Solid Edge part; units mm, degrees
sketch "Sketch1" plane through (0, 0, 0) normal (0, 0, -1) x (-1, 0, 0)
  line L0 (-66.5566, 13.1686) -> (-55.0566, 13.1686)
  line L1 (-55.0566, 13.1686) -> (-55.0566, 22.6686)
  line L2 (-55.0566, 22.6686) -> (-66.5566, 22.6686)
  line L3 (-66.5566, 22.6686) -> (-66.5566, 13.1686)
  line L4 (-51.5566, 13.1686) -> (-40.0566, 13.1686)
  line L5 (-40.0566, 13.1686) -> (-40.0566, 22.6686)
  line L6 (-40.0566, 22.6686) -> (-51.5566, 22.6686)
  line L7 (-51.5566, 22.6686) -> (-51.5566, 13.1686)
  line L8 (-32.5566, 10.1686) -> (-18.5566, 10.1686)
  line L9 (-18.5566, 10.1686) -> (-18.5566, 22.6686)
  line L10 (-18.5566, 22.6686) -> (-36.5566, 22.6686)
  line L11 (-36.5566, 22.6686) -> (-36.5566, 12.1686)
  line L12 (-32.5566, 10.1686) -> (-36.5566, 12.1686)
  line L13 (-92.5566, 26.1578) -> (-21.5566, 26.1578)
  line L14 (-21.5566, 26.1578) -> (-15.0566, 29.1686)
  line L15 (-15.0566, 29.1686) -> (-0.0566, 29.1686)
  line L16 (-0.0566, 29.1686) -> (-0.0566, 23.1686)
  line L17 (-15.0566, 23.1686) -> (-0.0566, 23.1686)
  line L18 (-15.0566, 23.1686) -> (-15.0566, 12.6686)
  line L19 (-15.0566, 12.6686) -> (-0.0566, 12.6686)
  line L20 (-0.0566, 12.6686) -> (-0.0566, 2.6686)
  line L21 (-26.2997, 2.6686) -> (-0.0566, 2.6686)
  line L22 (-40.1546, 9.1578) -> (-26.2997, 2.6686)
  line L23 (-65.1546, 9.1578) -> (-40.1546, 9.1578)
  line L24 (-77.5566, -0.3422) -> (-65.1546, 9.1578)
  line L25 (-92.5566, -0.3422) -> (-77.5566, -0.3422)
  line L26 (-92.5566, 3.6578) -> (-92.5566, -0.3422)
  line L27 (-92.5566, 3.6578) -> (-78.5566, 3.6578)
  line L28 (-78.5566, 3.6578) -> (-71.5566, 9.1578)
  line L29 (-92.5566, 9.1578) -> (-71.5566, 9.1578)
  line L30 (-92.5566, 9.1578) -> (-92.5566, 13.1578)
  line L31 (-92.5566, 13.1578) -> (-70.0566, 13.1578)
  line L32 (-70.0566, 13.1578) -> (-70.0566, 22.1578)
  line L33 (-92.5566, 22.1578) -> (-70.0566, 22.1578)
  line L34 (-92.5566, 22.1578) -> (-92.5566, 26.1578)
  dimension "D1" = 0.0566
  dimension "D2" = 15.0566
  dimension "D3" = 15.0566
  dimension "D4" = 0.0566
  dimension "D5" = 92.5566
  dimension "D6" = 66.5566
  dimension "D7" = 55.0566
  dimension "D8" = 70.0566
  dimension "D9" = 92.5566
  dimension "D10" = 92.5566
  dimension "D11" = 92.5566
  dimension "D12" = 40.1546
  dimension "D13" = 32.5566
  dimension "D14" = 18.5566
  dimension "D15" = 18.5566
  dimension "D16" = 36.5566
  dimension "D17" = 32.5566
  dimension "D18" = 92.5566
  dimension "D19" = 15.0566
  dimension "D20" = 26.2997
  dimension "D21" = 65.1546
  dimension "D22" = 92.5566
  dimension "D23" = 92.5566
  dimension "D24" = 92.5566
  dimension "D25" = 77.5566
extrude "Protrusion1" add sketch "Sketch1" against normal blind 15.0368
sketch "Sketch2" plane through (13.1782, 2.6686, 7.5184) normal (0, -1, 0) x (1, 0, 0)
  line L0 (74.2537, 1.7409) -> (1.8784, 6.3912)
extrude "Enlèvement_matière_1" cut sketch "Sketch2" along normal mid plane 64.6684 material side at (51.2475, 2.6686, 11.6343)
sketch "Sketch3" plane through (7.6241, 29.1686, 7.4367) normal (0, 1, 0) x (-1, 0, 0)
  circle A0 centre (0.0398, 0.1367) radius 2.0955
  circle A1 centre (-79.9299, -2.362) radius 2.1098
extrude "Enlèvement_matière_3" cut sketch "Sketch3" along normal mid plane 246.888
fillet "Congé_1" radius 7.1911 4 edges at (0.0566, 26.1686, 14.8734) (0.0566, 7.6686, 14.8734) (0.0566, 26.1686, 0) (0.0566, 7.6686, 0)
fillet "Congé_2" radius 4.5761 6 edges at (92.5566, 1.6578, 8.93) (92.5566, 11.1578, 8.93) (92.5566, 24.1578, 8.93) (92.5566, 24.1578, 0) (92.5566, 11.1578, 0) (92.5566, 1.6578, 0)
fillet "Congé_3" radius 2.0593 15 edges at (15.0566, 23.1686, 6.9548) (15.0566, 12.6686, 6.9548) (36.5566, 22.6686, 6.2641) (36.5566, 12.1686, 6.2641) (32.5566, 10.1686, 6.3926) (18.5566, 10.1686, 6.8424) (18.5566, 22.6686, 6.8424) (40.0566, 13.1686, 6.1516) (40.0566, 22.6686, 6.1516) (51.5566, 22.6686, 5.7822) (55.0566, 13.1686, 5.6697) (51.5566, 13.1686, 5.7822) (55.0566, 22.6686, 5.6697) (66.5566, 22.6686, 5.3003) (66.5566, 13.1686, 5.3003)
fillet "Congé_5" radius 2.0593 2 edges at (70.0566, 13.1578, 5.1878) (70.0566, 22.1578, 5.1878)
fillet "Congé_6" radius 1.0296 2 edges at (71.5566, 9.1578, 5.1397) (78.5566, 3.6578, 4.9148)
fillet "Congé_7" radius 6.35 1 edges at (77.5566, -0.3422, 4.9469)
fillet "Congé_8" radius 6.35 5 edges at (40.1546, 9.1578, 6.1485) (65.1546, 9.1578, 5.3453) (26.2997, 2.6686, 6.5936) (15.0566, 29.1686, 6.9548) (21.5566, 26.1578, 6.746)
sketch "Sketch4" plane through (12.4715, 2.6686, 7.1983) normal (0, -1, 0) x (1, 0, 0)
  line L0 (-4.4993, -3.3547) -> (9.8456, -1.8628)
  line L1 (-4.03, 4.0259) -> (9.569, 2.6247)
  arc A0 (-4.03, 4.0259) -> (-4.4993, -3.3547) centre (-4.8872, 0.3752) ccw
  arc A1 (9.8456, -1.8628) -> (9.569, 2.6247) centre (9.6128, 0.3752) ccw
extrude "Enlèvement_matière_4" cut sketch "Sketch4" against normal blind 5.498
properties part number "AC_1.04"
Design review of the part built by this model. Coordinates are the model's own, in mm. A direction names the side the tool comes from. Coordinates: 2 decimals unless noted, no trailing zeros. Loops run counter-clockwise (first coordinate to the right, second up) from the corner with the lowest first, then second, coordinate; pieces in that order, holes last.
Item 1: Clearance check with flat-ended pins moving along their axes: pin 1 (6 mm diameter, centred on x = 80.5, z = 10, fed in from +Y); pin 2 (3.5 mm diameter, centred on x = 47, z = 5, fed in from -Y); pin 3 (1.5 mm diameter, centred on y = 17, z = 7.5, fed in from +X). State where each tip first meets the part, or that it passes through.
Completed:
pin 1: stops at y = 26.16
pin 2: stops at y = 9.16
pin 3: stops at x = 70.06
Item 2: Add section A-A (y = 6.5). Give the number of separate pieces and of enclosed holes in the cut face, and give its area (3 significant figures).
Completed:
separate pieces: 2
enclosed holes: 1
area: 398 mm2
Item 3: Add section D-D (x = 26). Write out the cut boundary in (y, z).
Completed:
outline: (2.77, 0) - (10.17, 0) - (10.17, 13.21) - (2.77, 13.21) - close; (22.67, 0) - (26.16, 0) - (26.16, 13.21) - (22.67, 13.21) - close
Item 4: Add section C-C (x = 77). Write out the cut boundary in (y, z).
Completed:
outline: (0.26, 0) - (4.88, 0) - (4.88, 9.93) - (0.26, 9.93) - close; (9.16, 0) - (13.16, 0) - (13.16, 9.93) - (9.16, 9.93) - close; (22.16, 0) - (26.16, 0) - (26.16, 9.93) - (22.16, 9.93) - close
Item 5: Wall thickness on L1, parallel to X at y = 15.75, z = 9.5; L2, parallel to Y at x = 87.5, z = 1; L3, parallel to X at y = 21.75, z = 10.25: over which ranges is each line inside the solid? List them lowest first.
Completed:
L1: x = 15.06 to 18.56, 36.56 to 40.06, 51.56 to 55.06, 66.56 to 70.06
L2: y = -0.34 to 3.66, 9.16 to 13.16, 22.16 to 26.16
L3: x = 14.95 to 18.9, 36.21 to 40.4, 51.21 to 55.4, 66.21 to 70.89
Item 6: For faces 1 (the flat face through (13, 2.669, 4)), 2 (the cylindrical face through (14.47, 22.55, 7.12)), 3 (the cylindrical face through (65.1, 8.8, 5.5)), 4 (the cylindrical face through (50.94, 13.76, 5.93)), list the 3-axis set-ups (+Z, -Z, +X, -X, +Y, -Y) from which the entire face can be reached by the end or side of a thin tool; tool diameter is ignored.
Completed:
face 1: +Z, -Z, -X, -Y
face 2: +Z, -Z, -X
face 3: +Z, -Z, -Y
face 4: +Z, -Z
Item 7: Add section B-B (x = 62). Write out the cut boundary in (y, z).
Completed:
outline: (9.16, 0) - (13.17, 0) - (13.17, 10.89) - (9.16, 10.89) - close; (22.67, 0) - (26.16, 0) - (26.16, 10.89) - (22.67, 10.89) - close
Item 8: Draft analysis for pull direction Y (two halves, no side actions). For faces 5 (the flat face through (46, 22.669, 6)), 6 (the flat face through (52, 9.158, 6)), 7 (the cylindrical face through (73.566, 8.482, 5.148)), 8 (the flat face through (58, 26.158, 5)), state which applies: pulls with the +Y half, pulls with the -Y half, needs draft (parallel to the pull), parting line crosses it, or undercut.
Completed:
face 5: undercut
face 6: pulls with the -Y half
face 7: undercut
face 8: pulls with the +Y half
